Geometry check sheet. Reference: the model listing, model coordinates, mm. Give positions to 0.01 mm unless a question says otherwise; leave off trailing zeros. Order: outer loops, then holes, each group sorted by start corner. A loop starts at its lowest first (then second) coordinate and runs counter-clockwise, first axis right, second up. Notation, with made-up numbers: M 70.25,63.5 L 97.25,63.5 A10 cw 97.25,81.5 Z; hole C 16.5,20.5 d10. An arc over 180 degrees is marked long. One line per question, with ' | ' between items. Start each with the question number.
from build123d import *

# Parameters (mm, degrees)
BOSS_EXTRUDE1_DEPTH = 3.3
SKETCH2_R           = 1.05
SKETCH2_R_2         = 2.75
SKETCH2_R_3         = 1.375
CUT_EXTRUDE1_DEPTH  = 3.3
SKETCH3_R           = 1.9
CUT_EXTRUDE2_DEPTH  = 2.15
SKETCH6_R           = 2
CUT_EXTRUDE3_DEPTH  = 10


with BuildPart() as part:
    # Sketch1 → Boss-Extrude1 (new body)
    with BuildSketch(Plane(origin=(0, 0, 0), x_dir=(1, 0, 0), z_dir=(0, 1, 0))):
        with BuildLine():
            Line((-82.493420768, 57.400657923), (-42.038461538, 22.79802623))
            ThreePointArc((-42.038461538, 22.79802623), (-31.538461538, 0), (-42.038461538, -22.79802623))
            Line((-42.038461538, -22.79802623), (-82.493420768, -57.400657923))
            ThreePointArc((-82.493420768, -57.400657923), (-83.592762845, -71.5), (-69.493420768, -72.599342077))
            Line((-69.493420768, -72.599342077), (-19.5, -29.838109366))
            ThreePointArc((-19.5, -29.838109366), (0, -22.636135597), (19.5, -29.838109366))
            Line((19.5, -29.838109366), (69.493420768, -72.599342077))
            ThreePointArc((69.493420768, -72.599342077), (83.592762845, -71.5), (82.493420768, -57.400657923))
            Line((82.493420768, -57.400657923), (42.038461538, -22.79802623))
            ThreePointArc((42.038461538, -22.79802623), (31.538461538, 0), (42.038461538, 22.79802623))
            Line((42.038461538, 22.79802623), (82.493420768, 57.400657923))
            ThreePointArc((82.493420768, 57.400657923), (83.592762845, 71.5), (69.493420768, 72.599342077))
            Line((69.493420768, 72.599342077), (19.5, 29.838109366))
            ThreePointArc((19.5, 29.838109366), (0, 22.636135597), (-19.5, 29.838109366))
            Line((-19.5, 29.838109366), (-69.493420768, 72.599342077))
            ThreePointArc((-69.493420768, 72.599342077), (-83.592762845, 71.5), (-82.493420768, 57.400657923))
        make_face()
    extrude(amount=BOSS_EXTRUDE1_DEPTH)

    # Sketch2 → Cut-Extrude1 (cut)
    with BuildSketch(Plane(origin=(0, 3.3, 0), x_dir=(1, 0, 0), z_dir=(0, 1, 0))):
        with Locations(Location((-76.45983211, 70.981844236, 0), (0, 0, 270))):
            Circle(SKETCH2_R)
        with Locations(Location((-70.011576532, 65.466411342, 0), (0, 0, 270))):
            Circle(SKETCH2_R)
        with Locations(Location((-75.527009425, 59.018155764, 0), (0, 0, 270))):
            Circle(SKETCH2_R)
        with Locations(Location((-81.975265004, 64.533588658, 0), (0, 0, 270))):
            Circle(SKETCH2_R)
        with Locations(Location((75.527009425, 59.018155764, 0), (0, 0, 270))):
            Circle(SKETCH2_R)
        with Locations(Location((81.975265004, 64.533588658, 0), (0, 0, 270))):
            Circle(SKETCH2_R)
        with Locations(Location((76.45983211, 70.981844236, 0), (0, 0, 270))):
            Circle(SKETCH2_R)
        with Locations(Location((70.011576532, 65.466411342, 0), (0, 0, 270))):
            Circle(SKETCH2_R)
        with Locations(Location((-76.45983211, -70.981844236, 0), (0, 0, 270))):
            Circle(SKETCH2_R)
        with Locations(Location((-81.975265004, -64.533588658, 0), (0, 0, 270))):
            Circle(SKETCH2_R)
        with Locations(Location((-75.527009425, -59.018155764, 0), (0, 0, 270))):
            Circle(SKETCH2_R)
        with Locations(Location((-70.011576532, -65.466411342, 0), (0, 0, 270))):
            Circle(SKETCH2_R)
        with Locations(Location((70.011576532, -65.466411342, 0), (0, 0, 270))):
            Circle(SKETCH2_R)
        with Locations(Location((76.45983211, -70.981844236, 0), (0, 0, 270))):
            Circle(SKETCH2_R)
        with Locations(Location((81.975265004, -64.533588658, 0), (0, 0, 270))):
            Circle(SKETCH2_R)
        with Locations(Location((75.527009425, -59.018155764, 0), (0, 0, 270))):
            Circle(SKETCH2_R)
        with Locations(Location((-75.993420768, 65, 0), (0, 0, 270))):
            Circle(SKETCH2_R_2)
        with Locations(Location((75.993420768, 65, 0), (0, 0, 270))):
            Circle(SKETCH2_R_2)
        with Locations(Location((75.993420768, -65, 0), (0, 0, 270))):
            Circle(SKETCH2_R_2)
        with Locations(Location((-75.993420768, -65, 0), (0, 0, 270))):
            Circle(SKETCH2_R_2)
        with Locations(Location((-24, 16.5, 0), (0, 0, 270))):
            Circle(SKETCH2_R_3)
        with Locations(Location((24, 16.5, 0), (0, 0, 270))):
            Circle(SKETCH2_R_3)
        with Locations(Location((24, -16.5, 0), (0, 0, 270))):
            Circle(SKETCH2_R_3)
        with Locations(Location((-24, -16.5, 0), (0, 0, 270))):
            Circle(SKETCH2_R_3)
    extrude(amount=-CUT_EXTRUDE1_DEPTH, mode=Mode.SUBTRACT)

    # Sketch3 → Cut-Extrude2 (cut)
    with BuildSketch(Plane.XZ):
        with Locations(Location((-76.45983211, 70.981844236, 0), (0, 0, 270))):
            Circle(SKETCH3_R)
        with Locations(Location((-70.011576532, 65.466411342, 0), (0, 0, 270))):
            Circle(SKETCH3_R)
        with Locations(Location((-75.527009425, 59.018155764, 0), (0, 0, 270))):
            Circle(SKETCH3_R)
        with Locations(Location((-81.975265004, 64.533588658, 0), (0, 0, 270))):
            Circle(SKETCH3_R)
        with Locations(Location((81.975265004, 64.533588658, 0), (0, 0, 270))):
            Circle(SKETCH3_R)
        with Locations(Location((75.527009425, 59.018155764, 0), (0, 0, 270))):
            Circle(SKETCH3_R)
        with Locations(Location((70.011576532, 65.466411342, 0), (0, 0, 270))):
            Circle(SKETCH3_R)
        with Locations(Location((76.45983211, 70.981844236, 0), (0, 0, 270))):
            Circle(SKETCH3_R)
        with Locations(Location((76.45983211, -70.981844236, 0), (0, 0, 270))):
            Circle(SKETCH3_R)
        with Locations(Location((70.011576532, -65.466411342, 0), (0, 0, 270))):
            Circle(SKETCH3_R)
        with Locations(Location((75.527009425, -59.018155764, 0), (0, 0, 270))):
            Circle(SKETCH3_R)
        with Locations(Location((81.975265004, -64.533588658, 0), (0, 0, 270))):
            Circle(SKETCH3_R)
        with Locations(Location((-81.975265004, -64.533588658, 0), (0, 0, 270))):
            Circle(SKETCH3_R)
        with Locations(Location((-75.527009425, -59.018155764, 0), (0, 0, 270))):
            Circle(SKETCH3_R)
        with Locations(Location((-70.011576532, -65.466411342, 0), (0, 0, 270))):
            Circle(SKETCH3_R)
        with Locations(Location((-76.45983211, -70.981844236, 0), (0, 0, 270))):
            Circle(SKETCH3_R)
    extrude(amount=-CUT_EXTRUDE2_DEPTH, mode=Mode.SUBTRACT)

    # Sketch6 → Cut-Extrude3 (cut)
    with BuildSketch(Plane(origin=(0, 3.3, 0), x_dir=(1, 0, 0), z_dir=(0, 1, 0))):
        with Locations(Location((-15.25, 15.25, 0), (0, 0, 270))):
            Circle(SKETCH6_R)
        with Locations(Location((15.25, 15.25, 0), (0, 0, 270))):
            Circle(SKETCH6_R)
        with Locations(Location((15.25, -15.25, 0), (0, 0, 270))):
            Circle(SKETCH6_R)
        with Locations(Location((-15.25, -15.25, 0), (0, 0, 270))):
            Circle(SKETCH6_R)
        with BuildLine():
            Line((-20.5, 9), (-20.5, -9))
            ThreePointArc((-20.5, -9), (-19.767766953, -10.767766953), (-18, -11.5))
            ThreePointArc((-18, -11.5), (-13.775017592, 0), (-18, 11.5))
            ThreePointArc((-18, 11.5), (-19.767766953, 10.767766953), (-20.5, 9))
        make_face()
        with BuildLine():
            Line((20.5, 9), (20.5, -9))
            ThreePointArc((20.5, -9), (19.767766953, -10.767766953), (18, -11.5))
            ThreePointArc((18, -11.5), (13.775017592, 0), (18, 11.5))
            ThreePointArc((18, 11.5), (19.767766953, 10.767766953), (20.5, 9))
        make_face()
    extrude(amount=-CUT_EXTRUDE3_DEPTH, mode=Mode.SUBTRACT)


solid = part.part
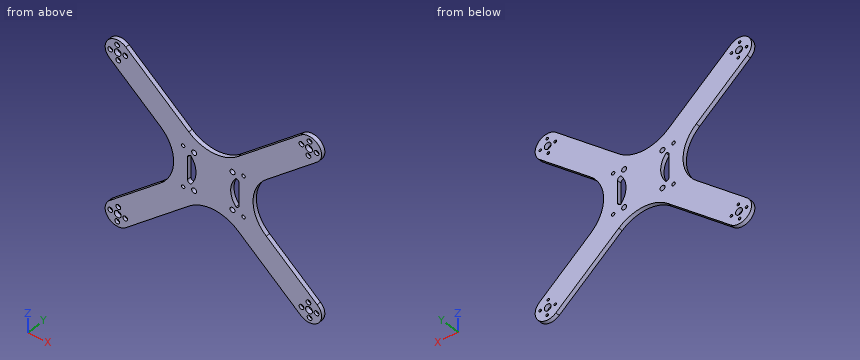
Item 1: Cross-section at D-D, the plane x = -1. Record the cut outline in (y, z), plus the area to 3 significant figures.
Item 2: Depth check by flat-ended pin: pin 1 (1.7 mm diameter, centred on x = -76.46, z = 70.98, fed in from +Y). Enter the tip coordinate at first touch or a pass-through.
Item 3: Material ranges on line 1 along Z through (x, y) = (-71.5, 0.4); line 2 along X through (y, z) = (1.9, 3); line 3 along X through (y, z) = (0.85, -14.5), recorded low to high.
Item 4: Cross-section at B-B, the plane x = 52. Record the cut outline in (y, z).
Item 5: Cross-section at A-A, the plane z = 0. Record the cut outline in (x, y).
Item 6: Cross-section at C-C, the plane y = 0.6. State how many separate pieces and enclosed holes the cut face has, plus the area to 3 significant figures.
Outcome:
1) outline: M 0,-22.65 L 3.3,-22.65 L 3.3,22.65 L 0,22.65 Z | area: 150 mm²
2) pin 1: passes through
3) line 1: z = -73.93 to -66.65, -64.29 to -48, 48 to 64.29, 66.65 to 73.93 | line 2: x = -31.69 to -20.5, -14.03 to 14.03, 20.5 to 31.69 | line 3: x = -35.28 to -17.1, -13.4 to 13.4, 17.1 to 35.28
4) outline: M 0,-57.64 L 3.3,-57.64 L 3.3,-31.32 L 0,-31.32 Z; M 0,31.32 L 3.3,31.32 L 3.3,57.64 L 0,57.64 Z
5) outline: M -31.54,0 L -20.5,0 L -20.5,3.3 L -31.54,3.3 Z; M -13.78,0 L 13.78,0 L 13.78,3.3 L -13.78,3.3 Z; M 20.5,0 L 31.54,0 L 31.54,3.3 L 20.5,3.3 Z
6) separate pieces: 1 | enclosed holes: 30 | area: 8,450 mm²
